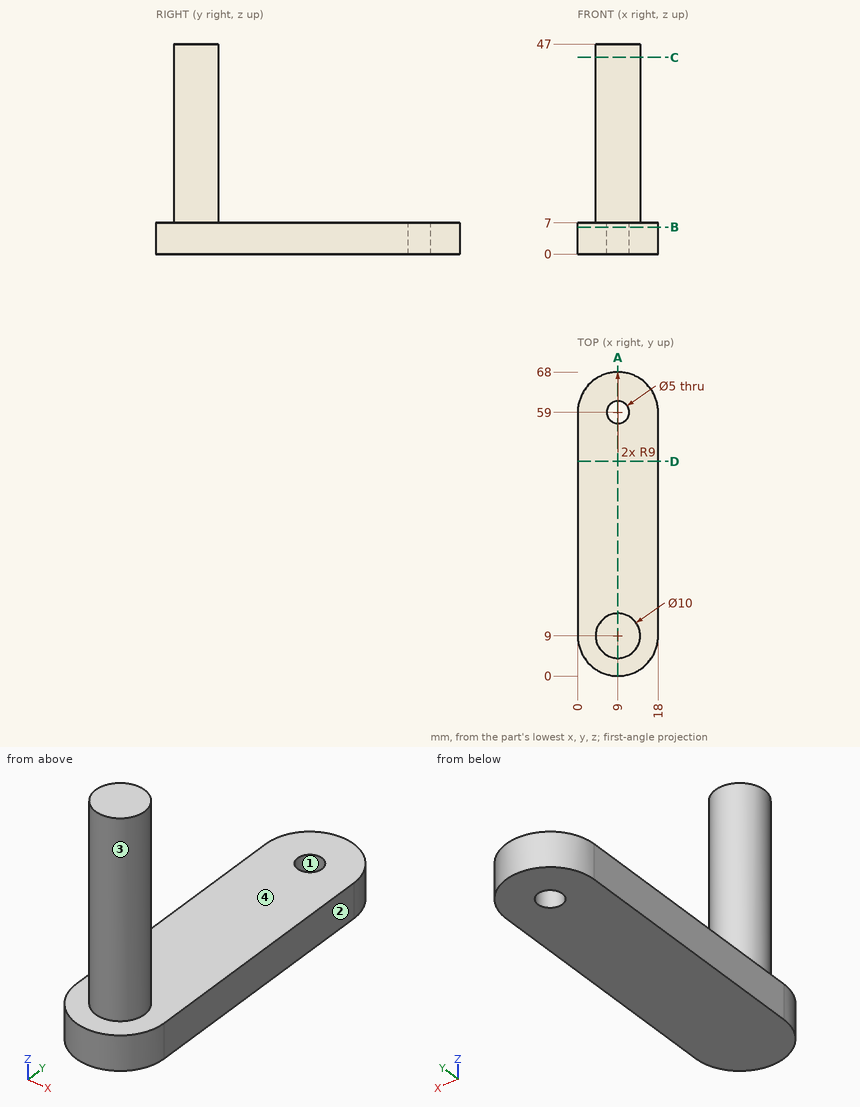
Study the drawing (mm; zero at the part's minimum x, y, z) and answer. Round coordinates to 2 decimals unless told otherwise and drop trailing zeros. Loops run counter-clockwise (first coordinate to the right, second up) from the corner with the lowest first, then second, coordinate; pieces in that order, holes last. Notation, with made-up numbers: (-35.5, 42.5) -> (-29.5, 42.5) arc R37 ccw to (-29.5, 79.5) -> close; hole circle Ø11 at (7, 10). An arc over 180 degrees is marked (long way). One line per item, written item: value.
1) A cutting plane is placed at D-D (y = 48). Determine the outline of the cut face in (x, z).
Answer list:
outline: (0, 0) -> (18, 0) -> (18, 7) -> (0, 7) -> close
2) Flat-ended cylindrical pins translate along their axes: P1, Ø3, axis at x = 8, z = 10, coming from the +Y side; P2, Ø1.5, axis at x = 4, z = 39, coming from the +Y side; P3, Ø9, axis at x = 8.5, y = 32, coming from the +Z side. Find the tip coordinate at first contact, or state that the pin passes through.
Answer list:
P1: stops at y = 14
P2: stops at y = 11.63
P3: stops at z = 7
3) A cutting plane is placed at B-B (z = 6). Determine the outline of the cut face in (x, y).
Answer list:
outline: (0, 9) arc R9 ccw to (18, 9) -> (18, 59) arc R9 ccw to (0, 59) -> close; hole circle Ø5 at (9, 59)
4) A cutting plane is placed at C-C (z = 44). Determine the outline of the cut face in (x, y).
Answer list:
outline: circle Ø10 at (9, 9)
5) Consider L1, parallel to Y at x = 9, z = 4; L2, parallel to Z at x = 5.5, y = 57.5; L3, parallel to Y at x = 9, z = 13.5. Determine where each line is inside the solid, lowest interval first. Write a range as [from, to].
Answer list:
L1: y = [0, 56.5], [61.5, 68]
L2: z = [0, 7]
L3: y = [4, 14]
6) A cutting plane is placed at A-A (x = 9). Determine the outline of the cut face in (y, z), and give its area (3 significant figures).
Answer list:
outline: (0, 0) -> (56.5, 0) -> (56.5, 7) -> (14, 7) -> (14, 47) -> (4, 47) -> (4, 7) -> (0, 7) -> close; (61.5, 0) -> (68, 0) -> (68, 7) -> (61.5, 7) -> close
area: 841 mm²
7) The mould has two halves that part along X. Classify the marked faces 1, 2, 3 and 4: pulls with the +X half, pulls with the -X half, needs draft (parallel to the pull), parting line crosses it, or undercut.
Answer list:
face 1: undercut
face 2: pulls with the +X half
face 3: parting line crosses it
face 4: needs draft
